Part model, mm, in its own coordinate system. Face numbers are marked on the shaded views. A direction names the side the tool comes from. Give positions to 0.01 mm unless a question says otherwise; leave off trailing zeros. Write each loop counter-clockwise with the first axis right and the second up, starting at its lowest first coordinate (ties: lowest second). Pieces come first, ordered by that corner, then holes.
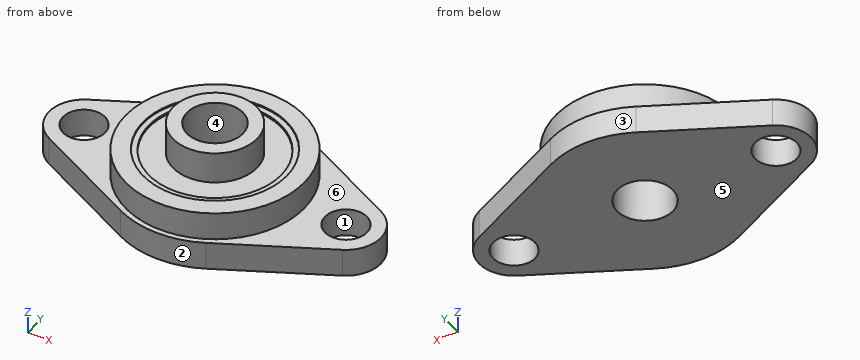
Autodesk Inventor part; units mm, degrees
ref_plane "YZ Plane" through (0, 0, 0) normal (1, 0, 0) x (0, 1, 0)
ref_plane "XZ Plane" through (0, 0, 0) normal (0, 1, 0) x (-1, 0, 0)
ref_plane "XY Plane" through (0, 0, 0) normal (0, 0, 1) x (1, 0, 0)
sketch "Szkic1" plane through (0, 0, 0) normal (0, 0, 1) x (1, 0, 0)
  arc A0 (21.0167, -4.4567) -> (21.0167, 4.4567) centre (18.75, 0) ccw
  arc A1 (-21.0167, 4.4567) -> (-21.0167, -4.4567) centre (-18.75, 0) ccw
  line L0 (6.12, -12.0331) -> (21.0167, -4.4567)
  line L1 (6.12, 12.0331) -> (21.0167, 4.4567)
  line L2 (-21.0167, 4.4567) -> (-6.12, 12.0331)
  line L3 (-21.0167, -4.4567) -> (-6.12, -12.0331)
  arc A2 (-6.12, -12.0331) -> (6.12, -12.0331) centre (0, 0) ccw
  arc A3 (6.12, 12.0331) -> (-6.12, 12.0331) centre (0, 0) ccw
  dimension "d3" = 10
  dimension "d4" = 10
  dimension "d5" = 37.5
  dimension "d6" = 18.75
  dimension "d7" = 0
extrude "Wyciągnięcie proste1" add sketch "Szkic1" along normal blind 4
sketch "Szkic2" plane through (0, 0, 4) normal (0, 0, 1) x (1, 0, 0)
  arc A0 (-21.0167, 4.4567) -> (-21.0167, -4.4567) centre (-18.75, 0) ccw
  line L0 (6.12, -12.0331) -> (21.0167, -4.4567)
  arc A1 (21.0167, -4.4567) -> (21.0167, 4.4567) centre (18.75, 0) ccw
  line L1 (21.0167, 4.4567) -> (6.12, 12.0331)
  arc A2 (6.12, 12.0331) -> (-6.12, 12.0331) centre (0, 0) ccw
  line L2 (-6.12, 12.0331) -> (-21.0167, 4.4567)
  arc A3 (-21.0167, 4.4567) -> (-21.0167, -4.4567) centre (-18.75, 0) ccw
  line L3 (-21.0167, -4.4567) -> (-6.12, -12.0331)
  arc A4 (-6.12, -12.0331) -> (6.12, -12.0331) centre (0, 0) ccw
  circle A5 centre (0, 0) radius 12.75
  dimension "d10" = 25.5
extrude "Wyciągnięcie proste2" add sketch "Szkic2" along normal blind 4 contours A5
hole "Otwór1" at (18.75, 0, 4) at (-18.75, 0, 4) direction (0, 0, -1) diameter 6 end through all
sketch "Szkic3" plane through (0, 0, 8) normal (0, 0, 1) x (1, 0, 0)
  circle A0 centre (0, 0) radius 10.25
  circle A1 centre (0, 0) radius 9.45
  circle A2 centre (0, 0) radius 6
  circle A3 centre (0, 0) radius 4
  dimension "d20" = 20.5
  dimension "d21" = 0.8
  dimension "d22" = 12
  dimension "d23" = 2
extrude "Wyciągnięcie proste3" cut sketch "Szkic3" against normal blind 0.2 contours A0
extrude "Wyciągnięcie proste4" cut sketch "Szkic3" against normal blind 0.5 contours A1
extrude "Wyciągnięcie proste5" cut sketch "Szkic3" against normal up to surface (8 mm away) contours A3
extrude "Wyciągnięcie proste6" add sketch "Szkic3" along normal blind 4 contours A2
properties part number "COTS_GENERIC_8mm_Dia_Ball_Screw_Top_Bearing_Block" material "Tworzywo sztuczne LCP"
1) Saw through at A-A, the plane y = 0. Count the separate pieces of the cut face and the enclosed holes in it, then the cut area to 3 significant figures.
Answers follow:
separate pieces: 4
enclosed holes: 0
area: 192 mm2
2) Saw through at C-C, the plane x = 0. Write the cut outline in (y, z).
Answers follow:
outline: (-13.5, 0) - (-4, 0) - (-4, 12) - (-6, 12) - (-6, 7.5) - (-9.45, 7.5) - (-9.45, 7.8) - (-10.25, 7.8) - (-10.25, 8) - (-12.75, 8) - (-12.75, 4) - (-13.5, 4) - close; (4, 0) - (13.5, 0) - (13.5, 4) - (12.75, 4) - (12.75, 8) - (10.25, 8) - (10.25, 7.8) - (9.45, 7.8) - (9.45, 7.5) - (6, 7.5) - (6, 12) - (4, 12) - close
3) Saw through at D-D, the plane y = -3.5. Write the cut outline in (x, z), then the cut area to 3 significant figures.
Answers follow:
outline: (-22.32, 0) - (-1.94, 0) - (-1.94, 12) - (-4.87, 12) - (-4.87, 7.5) - (-8.78, 7.5) - (-8.78, 7.8) - (-9.63, 7.8) - (-9.63, 8) - (-12.26, 8) - (-12.26, 4) - (-22.32, 4) - close; (1.94, 0) - (22.32, 0) - (22.32, 4) - (12.26, 4) - (12.26, 8) - (9.63, 8) - (9.63, 7.8) - (8.78, 7.8) - (8.78, 7.5) - (4.87, 7.5) - (4.87, 12) - (1.94, 12) - close
area: 265 mm2
4) Two-plate mould, pull along Y, no slides. Class the marked faces 1, 2, 3 and 4: +Y half, -Y half, draft (parallel to the pull), parting line (faces both ways), or undercut.
Answers follow:
face 1: undercut
face 2: -Y half
face 3: +Y half
face 4: undercut
5) 3-axis set-ups, long thin cutter, end or side, ignore diameter. For the marked faces 5 and 6: which of +Z, -Z, +X, -X, +Y, -Y reach the whole face in a straight line?
Answers follow:
face 5: -Z, +X, -X, +Y, -Y
face 6: +Z
6) Wall check: L1, parallel to Y at x = 0, z = 7.9; L2, parallel to Z at x = -12, y = 2; L3, parallel to Z at x = -3.5, y = 6.5. Give the ranges that are in metal, low to high.
Answers follow:
L1: y = -12.75 to -10.25, -6 to -4, 4 to 6, 10.25 to 12.75
L2: z = 0 to 8
L3: z = 0 to 7.5
7) Saw through at B-B, the plane z = 3.5. Write the cut outline in (x, y).
Answers follow:
outline: (-21.02, -4.46) - (-6.12, -12.03) arc R13.5 ccw to (6.12, -12.03) - (21.02, -4.46) arc R5 ccw to (21.02, 4.46) - (6.12, 12.03) arc R13.5 ccw to (-6.12, 12.03) - (-21.02, 4.46) arc R5 ccw to start; hole circle Ø6 at (-18.75, 0); hole circle Ø8 at (0, 0); hole circle Ø6 at (18.75, 0)
8) Pin check, flat tips, straight feed: pin 1 Ø2 at (x, y) = (6, -7) entering from +Z; pin 2 Ø1 at (y, z) = (-6, 10) entering from -X. Stop position of each tip, or through.
Answers follow:
pin 1: stops at z = 7.8
pin 2: stops at x = -2.4
